For this review, take the finished solid that the model builds, in its own axes (mm). Face numbers are marked on the shaded views. Give positions to 0.01 mm unless a question says otherwise; leave off trailing zeros. Loops run counter-clockwise (first coordinate to the right, second up) from the corner with the lowest first, then second, coordinate; pieces in that order, holes last. Notation, with made-up numbers: M 54,69 L 71,69 A31 ccw 71,108 Z; hole C 29.25,59 d6. An arc over 180 degrees is marked long. Use CSV: the item, a comma, the result in double quotes. Start each with the question number.
1. Take a section at D-D, the plane x = -1.5. Write out the cut boundary in (y, z).
2. Take a section at C-C, the plane y = 31. Write out the cut boundary in (x, z) (1 decimal), and give its area (3 significant figures).
3. The part is to be moulded in two halves that separate along Y. For the marked faces 1, 2, 3 and 4, say which applies: pulls with the +Y half, pulls with the -Y half, needs draft (parallel to the pull), parting line crosses it, or undercut.
4. Insertion check: P1, Ø4, axis at y = 18, z = 8, coming from the +X side. The pin has a flat end and moves straight along its axis. Give the tip position at first contact, or say it passes through.
5. Take a section at A-A, the plane x = -4.75. Write out the cut boundary in (y, z), and give its area (3 significant figures).
6. Take a section at B-B, the plane z = 8.75. State how many separate pieces and enclosed holes the cut face has, and give its area (3 significant figures).
7. To check wall thickness, follow line 1 (Y direction, x = -6.5, z = 8.75); line 2 (Y direction, x = -3, z = 10.25); line 3 (Z direction, x = -4.25, y = 31.5). State the ranges of each line that lie inside material, in increasing order. Write a range as [from, to].
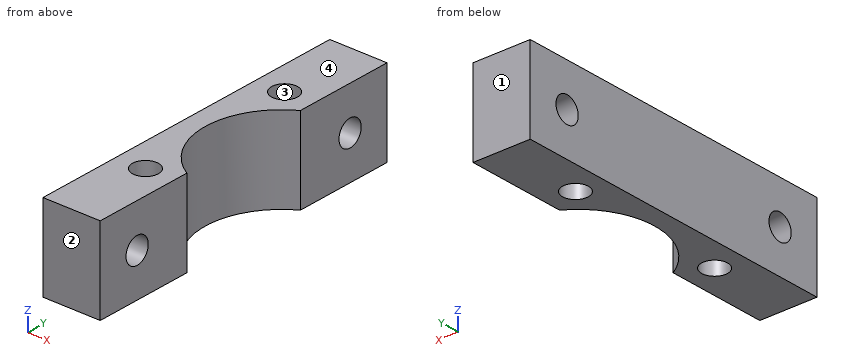
from build123d import *

# Parameters (mm, degrees)
F0_R     = 2.15265
F1_DEPTH = 14.2875
F2_R     = 2.15265
F3_DEPTH = 9.525


with BuildPart() as f1:
    # F0 (on Top) → F1 (new body)
    with BuildSketch(Plane.XY):
        with BuildLine():
            ThreePointArc((0, 0), (-6.35, 10.998523), (0, 21.997045))
            Line((0, 21.997045), (0, 38.756407))
            Line((0, 38.756407), (-9.525, 38.756407))
            Line((-9.525, 38.756407), (-9.525, -16.759362))
            Line((-9.525, -16.759362), (0, -16.759362))
            Line((0, -16.759362), (0, 0))
        make_face()
        with Locations((-4.7625, -2.471862)):
            Circle(F0_R, mode=Mode.SUBTRACT)
        with Locations((-4.7625, 24.468907)):
            Circle(F0_R, mode=Mode.SUBTRACT)
    extrude(amount=F1_DEPTH)

    # F2 (on face) → F3 (cut, through all)
    with BuildSketch(Plane(origin=(-9.525, 0, 0), x_dir=(0, -1, 0), z_dir=(-1, 0, 0))):
        with Locations((9.615612, 7.14375)):
            Circle(F2_R)
        with Locations((-31.612657, 7.14375)):
            Circle(F2_R)
    extrude(amount=-F3_DEPTH, mode=Mode.SUBTRACT)


solid = f1.part
Result set:
1,outline,"M -16.76,0 L 1.02,0 L 1.02,14.29 L -16.76,14.29 Z; M 20.98,0 L 38.76,0 L 38.76,14.29 L 20.98,14.29 Z; hole C -9.62,7.14 d4.31; hole C 31.61,7.14 d4.31"
2,outline,"M -9.5,0 L 0,0 L 0,5.1 L -9.5,5.1 Z; M -9.5,9.2 L 0,9.2 L 0,14.3 L -9.5,14.3 Z"
2,area,"96.8 mm2"
3,face 1,"pulls with the +Y half"
3,face 2,"pulls with the -Y half"
3,face 3,"undercut"
3,face 4,"needs draft"
4,P1,"x = -2.61"
5,outline,"M -16.76,0 L -4.62,0 L -4.62,14.29 L -16.76,14.29 Z; M -0.32,0 L 4.83,0 L 4.83,14.29 L -0.32,14.29 Z; M 17.17,0 L 22.32,0 L 22.32,14.29 L 17.17,14.29 Z; M 26.62,0 L 38.76,0 L 38.76,14.29 L 26.62,14.29 Z; hole C -9.62,7.14 d4.31; hole C 31.61,7.14 d4.31"
5,area,"465 mm2"
6,separate pieces,"3"
6,enclosed holes,"2"
6,area,"346 mm2"
7,line 1,"[-16.76, -11.05], [-8.18, -3.74], [-1.2, 23.2], [25.74, 30.18], [33.05, 38.76]"
7,line 2,"[-16.76, -3.71], [-1.24, 2.4], [19.59, 23.23], [25.7, 38.76]"
7,line 3,"[0, 4.99], [9.29, 14.29]"
